CAD build for the part. Positions are in the model's coordinates, mm. Face numbers are marked on the shaded views. A direction names the side the tool comes from. Give positions to 0.01 mm unless a question says otherwise; leave off trailing zeros. Write each loop counter-clockwise with the first axis right and the second up, starting at its lowest first coordinate (ties: lowest second). Pieces come first, ordered by that corner, then holes. Notation, with made-up numbers: (46.5, 5) - (86.5, 5) arc R33 ccw to (86.5, 40) - close; hole circle Ø7 at (3, -36.75). An arc over 180 degrees is marked (long way). Put each result on its own line as item: value. Start each with the question number.
1. Cut at A-A on x = 0. List the corners of the cut face in (y, z), and give its area (3 significant figures).
2. Cut at B-B on z = 0. List the corners of the cut face in (x, y), and give its area (3 significant figures).
3. Cut at C-C on z = -5.25. List the corners of the cut face in (x, y), and give its area (3 significant figures).
4. Wall check: line 1 (X direction, y = 0.8, z = 0); line 2 (Y direction, x = 4.5, z = -7.75); line 3 (X direction, y = 2.4, z = 4). Give the ranges that are in metal, low to high.
5. Drop flat-ended pins along their axis: pin 1 (1.5 mm diameter, centred on x = 4.95, z = 4.95, fed in from +Y); pin 2 (1 mm diameter, centred on x = -1, y = 0.5, fed in from +Z); pin 3 (1 mm diameter, centred on y = 4, z = 1, fed in from -X). Give the stop position or say it passes through.
6. Tool access for the marked faces 1 and 2: list every direction of +Z, -Z, +X, -X, +Y, -Y with a clear straight run to the whole face (end or side of a thin tool).
7. Cut at D-D on y = 4. List the corners of the cut face in (x, z).
8. Mould opens along Z. For the marked faces 3, 4 and 5 say: +Z half, -Z half, draft (parallel to the pull), parting line (faces both ways), or undercut.
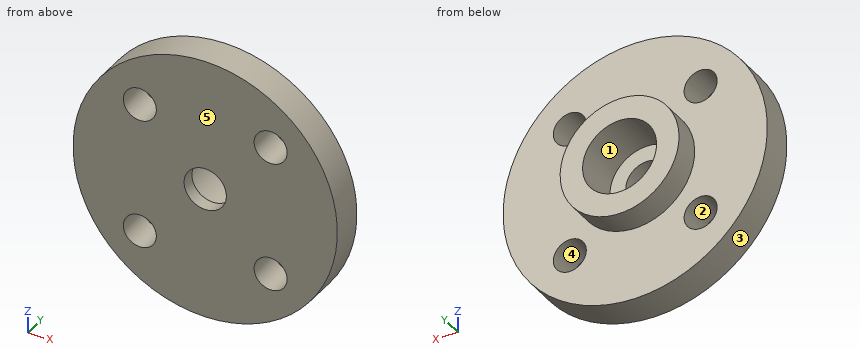
from build123d import *

# Parameters (mm, degrees)
ESQUISSE1_R                               = 10
ESQUISSE1_R_2                             = 1.6
BOSS_EXTRU_1_DEPTH                        = 2.5
ESQUISSE2_R                               = 4.5
ESQUISSE2_R_2                             = 2.8
BOSS_EXTRU_2_DEPTH                        = 2
TROU_POUR_TARAUDAGE_POUR_TROU_TARAUD_M3_D = 2.5
ENL_V_START                               = -1.5
ESQUISSE5_R                               = 2.8
ESQUISSE5_R_2                             = 1.6
ENL_V_MAT_EXTRU_1_DEPTH                   = 1.5


with BuildPart() as part:
    # Esquisse1 → Boss.-Extru.1 (new body)
    with BuildSketch(Plane(origin=(0, 0, 0), x_dir=(1, 0, 0), z_dir=(0, 1, 0))):
        with Locations(Location((0, 0, 0), (0, 0, 270))):
            Circle(ESQUISSE1_R)
        with Locations(Location((0, 0, 0), (0, 0, 270))):
            Circle(ESQUISSE1_R_2, mode=Mode.SUBTRACT)
    extrude(amount=BOSS_EXTRU_1_DEPTH)

    # Esquisse2 → Boss.-Extru.2 (add)
    with BuildSketch(Plane(origin=(0, 2.5, 0), x_dir=(1, 0, 0), z_dir=(0, 1, 0))):
        with Locations(Location((0, 0, 0), (0, 0, 270))):
            Circle(ESQUISSE2_R)
        with Locations(Location((0, 0, 0), (0, 0, 270))):
            Circle(ESQUISSE2_R_2, mode=Mode.SUBTRACT)
    extrude(amount=BOSS_EXTRU_2_DEPTH)

    # Trou pour taraudage pour trou taraudé M31 (through all)
    with Locations(Plane(origin=(0, 2.5, 0), x_dir=(1, 0, 0), z_dir=(0, 1, 0))):
        with Locations((4.949747468, -4.949747468), (-4.949747468, -4.949747468), (-4.949747468, 4.949747468), (4.949747468, 4.949747468)):
            Hole(TROU_POUR_TARAUDAGE_POUR_TROU_TARAUD_M3_D / 2)

    # Esquisse5 → Enlèv. mat.-Extru.1 (cut)
    with BuildSketch(Plane(origin=(0, 2.5, 0), x_dir=(1, 0, 0), z_dir=(0, 1, 0)).offset(ENL_V_START)):
        with Locations(Location((0, 0, 0), (0, 0, 270))):
            Circle(ESQUISSE5_R)
        with Locations(Location((0, 0, 0), (0, 0, 270))):
            Circle(ESQUISSE5_R_2, mode=Mode.SUBTRACT)
    extrude(amount=ENL_V_MAT_EXTRU_1_DEPTH, mode=Mode.SUBTRACT)


solid = part.part
Report:
1. outline: (0, -10) - (2.5, -10) - (2.5, -4.5) - (4.5, -4.5) - (4.5, -2.8) - (1, -2.8) - (1, -1.6) - (0, -1.6) - close; (0, 1.6) - (1, 1.6) - (1, 2.8) - (4.5, 2.8) - (4.5, 4.5) - (2.5, 4.5) - (2.5, 10) - (0, 10) - close
1. area: 45.2 mm²
2. outline: (-10, 0) - (-1.6, 0) - (-1.6, 1) - (-2.8, 1) - (-2.8, 4.5) - (-4.5, 4.5) - (-4.5, 2.5) - (-10, 2.5) - close; (1.6, 0) - (10, 0) - (10, 2.5) - (4.5, 2.5) - (4.5, 4.5) - (2.8, 4.5) - (2.8, 1) - (1.6, 1) - close
2. area: 45.2 mm²
3. outline: (-8.51, 0) - (-6.16, 0) - (-6.16, 2.5) - (-8.51, 2.5) - close; (-3.74, 0) - (3.74, 0) - (3.74, 2.5) - (-3.74, 2.5) - close; (6.16, 0) - (8.51, 0) - (8.51, 2.5) - (6.16, 2.5) - close
3. area: 30.4 mm²
4. line 1: x = -10 to -1.6, 1.6 to 10
4. line 2: y = 0 to 2.5
4. line 3: x = -9.17 to -5.76, -4.14 to 4.14, 5.76 to 9.17
5. pin 1: passes through
5. pin 2: stops at z = 9.99
5. pin 3: stops at x = -4.47
6. face 1: +Y
6. face 2: +Y, -Y
7. outline: circle Ø9 at (0, 0); hole circle Ø5.6 at (0, 0)
8. face 3: parting line
8. face 4: undercut
8. face 5: draft
